Read the model definition and answer for the solid it produces. Units are mm, in the model's axes. A direction names the side the tool comes from. Coordinates: 2 decimals unless noted, no trailing zeros. Loops run counter-clockwise (first coordinate to the right, second up) from the corner with the lowest first, then second, coordinate; pieces in that order, holes last.
Solid Edge part; units mm, degrees
sketch "Sketch1" plane through (0, 0, 0) normal (0, 0, 1) x (1, 0, 0)
  circle A0 centre (0, 0) radius 4.7625
extrude "Protrusion1" add sketch "Sketch1" along normal blind 6.35
sketch "Sketch2" plane through (0, 0, 0) normal (0, 0, -1) x (1, 0, 0)
  circle A0 centre (0, 0) radius 3.175
extrude "Protrusion2" add sketch "Sketch2" along normal blind 19.05
sketch "Sketch3" plane through (0, 0, -19.05) normal (0, 0, -1) x (1, 0, 0)
  circle A0 centre (0, 0) radius 3.1747
extrude "Cutout1" cut sketch "Sketch3" against normal blind 19.0309 flip side to cut
chamfer "Chamfer_1" distance 0.4762 angle 45 1 edges at (-3.1747, 0, -19.05)
sketch "Sketch4" plane through (0, 0, 6.35) normal (0, 0, 1) x (1, 0, 0)
  line L0 (-1.3748, 2.3812) -> (1.3748, 2.3812)
  line L1 (2.7496, 0) -> (1.3748, 2.3812)
  line L2 (1.3748, -2.3812) -> (2.7496, 0)
  line L3 (-1.3748, -2.3812) -> (1.3748, -2.3812)
  line L4 (-2.7496, 0) -> (-1.3748, -2.3812)
  line L5 (-1.3748, 2.3812) -> (-2.7496, 0)
extrude "Cutout2" cut sketch "Sketch4" against normal blind 3.175
properties part number "118797_3" material "Stainless Steel, 304"
Item 1: Find the intervals of material crossed by line 1 along Z through (x, y) = (1.5, 0.75) (3 decimals); line 2 along Z through (x, y) = (1.75, 4); line 3 along Y through (x, z) = (-1.5, 4), in increasing order.
Numbers:
line 1: z = -19.05 to 3.175
line 2: z = 0 to 6.35
line 3: y = -4.52 to -2.16, 2.16 to 4.52
Item 2: A cutting plane is placed at C-C on z = -8.5. Determine the outline of the cut face in (x, y).
Numbers:
outline: circle Ø6.35 at (0, 0)
Item 3: Given pin 1 (0.8 mm diameter, centred on x = -0.5, z = 4.5, fed in from -Y); pin 2 (1.5 mm diameter, centred on x = 0.5, z = -3.5, fed in from +Y); pin 3 (1.5 mm diameter, centred on x = 3.5, y = 1, fed in from -Z); pin 4 (1.4 mm diameter, centred on x = 0.5, y = 1, fed in from +Z) (3 decimals), each flat-ended and moving along its own axis, determine where each tip first touches the part or whether it passes through.
Numbers:
pin 1: stops at y = -4.76
pin 2: stops at y = 3.17
pin 3: stops at z = -18.86
pin 4: stops at z = 3.175
Item 4: A cutting plane is placed at D-D on y = -3.5. Determine the outline of the cut face in (x, z), then the cut area to 3 significant figures.
Numbers:
outline: (-3.23, 0) - (3.23, 0) - (3.23, 6.35) - (-3.23, 6.35) - close
area: 41.0 mm2
Item 5: Which of the six approach directions +Z, -Z, +X, -X, +Y, -Y give full straight-line access (tool end or side, diameter ignored) to faces 1 (the face through (0, -2.381, 5)), 2 (the face through (2.93, 1.22, -9.43)), 3 (the face through (2, -2, 6.35))?
Numbers:
face 1: +Z
face 2: -Z
face 3: +Z, +X, -X, +Y, -Y
Item 6: A cutting plane is placed at A-A on z = 4.75. Determine the outline of the cut face in (x, y) (1 decimal).
Numbers:
outline: circle Ø9.5 at (0, 0); hole (-2.7, 0) - (-1.4, -2.4) - (1.4, -2.4) - (2.7, 0) - (1.4, 2.4) - (-1.4, 2.4) - close
Item 7: Determine the mould class of faces 4 (the face through (2.05, -1.21, 4.78)), 5 (the face through (0, 0, -19.05)), 6 (the face through (-3.78, 2.9, 3.13)), 7 (the face through (-2.072, -1.174, 4.785)) for opening direction X: released by +X, released by -X, zero draft, split by the parting line, or undercut.
Numbers:
face 4: undercut
face 5: zero draft
face 6: split by the parting line
face 7: undercut
